Input: part model. Units: mm. Frame: model coordinates. A direction names the side the tool comes from. Round coordinates to 2 decimals unless told otherwise and drop trailing zeros. Order: outer loops, then holes, each group sorted by start corner. A loop starts at its lowest first (then second) coordinate and runs counter-clockwise, first axis right, second up.
Item 1: First-contact query: pin 1 (3 mm diameter, centred on y = 3.175, z = 6.35, fed in from -X) (3 decimals); pin 2 (2.5 mm diameter, centred on y = 3.175, z = -6.35, fed in from -X); pin 3 (8 mm diameter, centred on x = 11, z = 5.5, fed in from -Y). Flat tips, straight axial feed; report the tip coordinate or a pass-through.
Item 2: Reachability of faces 4 (the cylindrical face through (-6.22, 2.28, 5.38)), 5 (the flat face through (-15.875, 3, 0)) from +Z, -Z, +X, -X, +Y, -Y: full face, straight path, thin tool, end or side. Return the list, or none.
Item 3: Mould query, pull axis Y, two halves, no side actions, for faces 1 (the cylindrical face through (0, 0, 0)), 2 (the conical face through (3.831, 3.035, 6.168)), 3 (the flat face through (15.875, 3, 0)). Classes: released by +Y, released by -Y, zero draft, split by the parting line, or undercut.
Item 4: Cut plane C-C on x = 6. Output: boundary loops of the cut face in (y, z) (3 decimals), then the cut area to 3 significant figures.
Item 5: Cut plane A-A on z = 0. Output: boundary loops of the cut face in (x, y) (3 decimals).
Item 6: Cut plane B-B on x = -14. Output: boundary loops of the cut face in (y, z) (3 decimals), then the cut area to 3 significant figures.
Item 7: Cut plane D-D on z = -9. Output: boundary loops of the cut face in (x, y) (3 decimals).
Item 8: Line query: L1, parallel to X at y = 3.5, z = 0 (3 decimals); L2, parallel to Z at x = -7, y = 4.25. Output: solid intervals per line, ascending.
Autodesk Inventor part; units mm, degrees
ref_plane "YZ Plane" through (0, 0, 0) normal (1, 0, 0) x (0, 1, 0)
ref_plane "XZ Plane" through (0, 0, 0) normal (0, 1, 0) x (-1, 0, 0)
ref_plane "XY Plane" through (0, 0, 0) normal (0, 0, 1) x (1, 0, 0)
sketch "Sketch1" plane through (0, 0, 0) normal (0, 1, 0) x (-1, 0, 0)
  line L0 (-15.875, 12.7) -> (15.875, 12.7)
  line L1 (15.875, 12.7) -> (15.875, -12.7)
  line L2 (15.875, -12.7) -> (-15.875, -12.7)
  line L3 (-15.875, -12.7) -> (-15.875, 12.7)
  line L4 (-15.875, 12.7) -> (15.875, -12.7) construction
  line L5 (15.875, 12.7) -> (-15.875, -12.7) construction
  point P0 (0, 0)
  dimension "d0" = 31.75
  dimension "d1" = 25.4
extrude "Extrusion1" add sketch "Sketch1" along normal blind 6.35
sketch "Sketch2" plane through (-15.875, 0, -12.7) normal (-1, 0, 0) x (0, 0, 1)
  line L0 (12.7, 0) -> (12.7, 6.35) construction
  line L1 (25.4, 6.35) -> (0, 6.35) construction
  line L2 (12.7, 3.175) -> (6.35, 3.175) construction
  line L3 (12.7, 3.175) -> (19.05, 3.175) construction
  dimension "d4" = 6.35
  dimension "d5" = 180
hole "Hole1" at (-15.875, 3.175, -6.35) at (-15.875, 3.175, 6.35) direction (1, 0, 0) diameter 2.6416 depth 19.05 tip angle 118
sketch "Sketch3" plane through (-15.875, 0, -12.7) normal (-1, 0, 0) x (0, 0, 1)
  line L0 (12.7, 0) -> (12.7, 98.425) construction
  line L1 (12.7, 0) -> (111.125, 0) construction
  circle A0 centre (12.7, 98.425) radius 98.425
  dimension "d14" = 98.425
  dimension "d15" = 90
  dimension "d16" = 196.85
extrude "Extrusion2" cut sketch "Sketch3" against normal up to surface (31.75 mm away) keep common part
sketch "Sketch4" plane through (0, 6.35, 0) normal (0, 1, 0) x (1, 0, 0)
  line L0 (-15.875, 12.7) -> (-15.875, -12.7) construction
  line L1 (-15.875, 0) -> (3.175, 0) construction
  line L2 (-15.875, 0) -> (3.175, 0) construction
  line L3 (3.175, 0) -> (13.335, 0) construction
  line L4 (3.175, 0) -> (13.335, 0) construction
  point P0 (0, 0)
  dimension "d19" = 19.05
  dimension "d20" = 0
  dimension "d21" = 10.16
  dimension "d22" = 0
hole "Hole2" at (13.335, 6.35, 0) at (3.175, 6.35, 0) direction (0, -1, 0) diameter 2.6416 depth 19.05 tip angle 118
properties part number "4K adapter" material "Copper"
From the geometry:
1. pin 1: stops at x = -15.875
1. pin 2: stops at x = 3.22
1. pin 3: stops at y = 0.01
2. face 4: -X
2. face 5: +Z, -Z, -X, +Y, -Y
3. face 1: released by -Y
3. face 2: undercut
3. face 3: zero draft
4. outline: (0.823, -12.7) - (6.35, -12.7) - (6.35, 12.7) - (0.823, 12.7) arc R98.425 ccw to start
4. area: 154 mm2
5. outline: (-15.875, 0) - (1.854, 0) - (1.854, 6.35) - (-15.875, 6.35) - close; (4.496, 0) - (12.014, 0) - (12.014, 6.35) - (4.496, 6.35) - close; (14.656, 0) - (15.875, 0) - (15.875, 6.35) - (14.656, 6.35) - close
6. outline: (0.823, -12.7) - (6.35, -12.7) - (6.35, 12.7) - (0.823, 12.7) arc R98.425 ccw to start; hole circle Ø2.642 at (3.175, -6.35); hole circle Ø2.642 at (3.175, 6.35)
6. area: 143 mm2
7. outline: (-15.875, 0.412) - (15.875, 0.412) - (15.875, 6.35) - (-15.875, 6.35) - close
8. L1: x = -15.875 to 1.854, 4.496 to 12.014, 14.656 to 15.875
8. L2: z = -12.7 to -7.12, -5.58 to 5.58, 7.12 to 12.7
